Verification items for the finished model (mm, model axes). A direction names the side the tool comes from. Coordinates: 2 decimals unless noted, no trailing zeros. Order: outer loops, then holes, each group sorted by start corner. A loop starts at its lowest first (then second) coordinate and runs counter-clockwise, first axis right, second up. Notation, with made-up numbers: M -39.75,38 L -5.75,38 A18 cw -5.75,68 Z; hole C 14.5,-9.5 d9. An arc over 180 degrees is marked long. Use one line per item in the form item = value. Start each with the question number.
```python
from build123d import *

# Parameters (mm, degrees)
SKETCH2_W           = 13.35
SKETCH2_H           = 37.95
SKETCH2_R           = 1.4
SKETCH2_R_2         = 1
BOSS_EXTRUDE1_DEPTH = 5
SKETCH3_R           = 2
CUT_EXTRUDE1_DEPTH  = 2
CUT_EXTRUDE2_DEPTH  = 6
FILLET1_R           = 2
CHAMFER1_SIZE       = 0.4


with BuildPart() as part:
    # Sketch2 → Boss-Extrude1 (new body)
    with BuildSketch(Plane(origin=(0, 0, 0), x_dir=(1, 0, 0), z_dir=(0, 1, 0))):
        Rectangle(SKETCH2_W, SKETCH2_H)
        with Locations((-3.675, 13.975)):
            Circle(SKETCH2_R, mode=Mode.SUBTRACT)
        with Locations((3.675, -13.975)):
            Circle(SKETCH2_R, mode=Mode.SUBTRACT)
        with Locations((0, 15.75)):
            Circle(SKETCH2_R_2, mode=Mode.SUBTRACT)
        with Locations((0, -15.75)):
            Circle(SKETCH2_R_2, mode=Mode.SUBTRACT)
    extrude(amount=BOSS_EXTRUDE1_DEPTH)

    # Sketch3 → Cut-Extrude1 (cut)
    with BuildSketch(Plane(origin=(0, 5, 0), x_dir=(1, 0, 0), z_dir=(0, 1, 0))):
        with Locations((0, 15.75)):
            Circle(SKETCH3_R)
        with Locations((0, -15.75)):
            Circle(SKETCH3_R)
    extrude(amount=-CUT_EXTRUDE1_DEPTH, mode=Mode.SUBTRACT)

    # Sketch4 → Cut-Extrude2 (cut, through all)
    with BuildSketch(Plane(origin=(0, 5, 0), x_dir=(1, 0, 0), z_dir=(0, 1, 0))):
        with BuildLine():
            Line((-6.675, 10.575), (-2, 10.575))
            ThreePointArc((-2, 10.575), (-0.585786438, 9.989213562), (0, 8.575))
            Line((0, 8.575), (0, -11.75))
            ThreePointArc((0, -11.75), (-2.828427125, -12.921572875), (-4, -15.75))
            Line((-4, -15.75), (-4, -18.975))
            Line((-4, -18.975), (-6.675, -18.975))
            Line((-6.675, -18.975), (-6.675, 10.575))
        make_face()
    extrude(amount=-CUT_EXTRUDE2_DEPTH, mode=Mode.SUBTRACT)

    # Fillet1
    fillet1_edges = [part.edges().sort_by_distance(p)[0] for p in [
        (-6.675, 2.5, -10.575),
        (-4, 2.5, 18.975),
        (-6.675, 2.5, -18.975),
        (6.675, 2.5, -18.975),
        (6.675, 2.5, 18.975),
    ]]
    fillet(fillet1_edges, radius=FILLET1_R)

    # Chamfer1
    chamfer1_edges = [part.edges().sort_by_distance(p)[0] for p in [
        (-3.3375, 0, -10.575),
        (-0.585786438, 0, -9.989213562),
        (0, 0, 1.5875),
        (-2.828427125, 0, 12.921572875),
        (-2.828427125, 5, 12.921572875),
        (0, 5, 1.5875),
        (-0.585786438, 5, -9.989213562),
        (-3.3375, 5, -10.575),
        (-6.675, 0, -14.775),
        (-6.675, 5, -14.775),
        (-4, 5, 16.3625),
        (1.3375, 5, 18.975),
        (6.675, 5, 0),
        (0, 5, -18.975),
        (-3.414213562, 5, 18.389213562),
        (6.089213562, 5, 18.389213562),
        (6.089213562, 5, -18.389213562),
        (-6.089213562, 5, -18.389213562),
        (-6.089213562, 5, -11.160786438),
        (0, 0, -18.975),
        (6.675, 0, 0),
        (1.3375, 0, 18.975),
        (-4, 0, 16.3625),
        (-3.414213562, 0, 18.389213562),
        (6.089213562, 0, 18.389213562),
        (6.089213562, 0, -18.389213562),
        (-6.089213562, 0, -18.389213562),
        (-6.089213562, 0, -11.160786438),
    ]]
    chamfer(chamfer1_edges, length=CHAMFER1_SIZE)


solid = part.part
```
1. Material ranges on line 1 along X through (y, z) = (2.6, -14) (3 decimals); line 2 along Z through (x, y) = (-3.25, 1.7) (3 decimals); line 3 along X through (y, z) = (1.7, -15.75) (3 decimals), recorded low to high.
2. Cross-section at B-B on y = 1.5. Enter the section's corners in (x, z) (3 decimals), and give its area (3 significant figures).
3. Cross-section at D-D on y = 3.5. Enter the section's corners in (x, z) (3 decimals), and give its area (3 significant figures).
4. Cross-section at A-A on z = -15.75. Enter the section's corners in (x, y) (3 decimals).
5. Tool access check on faces 5 (the cylindrical face through (-2.797, 2.529, 12.891)), 6 (the cylindrical face through (-3.399, 2.471, 18.405)), 7 (the conical face through (-0.526, 0.292, -10.082)). Record the directions out of +Z, -Z, +X, -X, +Y, -Y that give a thin tool (end or side, any length) a straight path to the whole face; none if there is none.
6. Cross-section at C-C on z = 4.5. Enter the section's corners in (x, y) (3 decimals).
7. Depth check by flat-ended pin: P1, Ø1.5, axis at x = -5.5, y = 1, coming from the +Z side; P2, Ø1, axis at x = -2, z = -10.5, coming from the +Y side; P3, Ø1.2, axis at x = 0.5, z = 15, coming from the +Y side; P4, Ø0.6, axis at y = 2, z = 16.5, coming from the -X side. Enter the tip coordinate at first touch or a pass-through.
8. Release check for a two-part mould opening along X. For faces 1 (the cylindrical face through (3.493, 2.465, 12.587)), 2 (the cylindrical face through (-0.26, 4.014, 13.767)), 3 (the flat face through (-3, 3, -10.575)), 4 (the flat face through (0, 3, 1)) record: pulls with the +X half, pulls with the -X half, needs draft (parallel to the pull), parting line crosses it, or undercut.
Final values:
q1.line_1 = -6.675 to -5.075, -2.275 to 6.675
q1.line_2 = -18.975 to -15.309, -12.641 to -10.575, 13.418 to 18.536
q1.line_3 = -6.675 to -1, 1 to 6.675
q2.outline = M -6.675,-16.975 A2 ccw -4.675,-18.975 L 4.675,-18.975 A2 ccw 6.675,-16.975 L 6.675,16.975 A2 ccw 4.675,18.975 L -2,18.975 A2 ccw -4,16.975 L -4,15.75 A4 ccw 0,11.75 L 0,-8.575 A2 cw -2,-10.575 L -4.675,-10.575 A2 ccw -6.675,-12.575 Z; hole C -3.675,-13.975 d2.8; hole C 0,-15.75 d2; hole C 0,15.75 d2; hole C 3.675,13.975 d2.8
q2.area = 313 mm2
q3.outline = M -6.675,-16.975 A2 ccw -4.675,-18.975 L 4.675,-18.975 A2 ccw 6.675,-16.975 L 6.675,16.975 A2 ccw 4.675,18.975 L -2,18.975 A2 ccw -4,16.975 L -4,15.75 A4 ccw 0,11.75 L 0,-8.575 A2 cw -2,-10.575 L -4.675,-10.575 A2 ccw -6.675,-12.575 Z; hole C -3.675,-13.975 d2.8; hole C 0,-15.75 d4; hole C 0,15.75 d4; hole C 3.675,13.975 d2.8
q3.area = 294 mm2
q4.outline = M -6.675,0.4 L -6.275,0 L -1,0 L -1,3 L -2,3 L -2,5 L -6.275,5 L -6.675,4.6 Z; M 1,0 L 6.275,0 L 6.675,0.4 L 6.675,4.6 L 6.275,5 L 2,5 L 2,3 L 1,3 Z
q5.face_5 = -X, +Y, -Y
q5.face_6 = +Z, -X, +Y, -Y
q5.face_7 = -X, -Y
q6.outline = M 0,0.4 L 0.4,0 L 6.275,0 L 6.675,0.4 L 6.675,4.6 L 6.275,5 L 0.4,5 L 0,4.6 Z
q7.P1 = -10.58
q7.P2 = 5
q7.P3 = 3
q7.P4 = -4
q8.face_1 = undercut
q8.face_2 = undercut
q8.face_3 = needs draft
q8.face_4 = pulls with the -X half
